Part print with two shaded views. Sizes in mm from the minimum x, y, z corner. A direction names the side the tool comes from. Coordinates: 2 decimals unless noted, no trailing zeros. Write each loop counter-clockwise with the first axis right and the second up, starting at its lowest first coordinate (ties: lowest second). Pieces come first, ordered by that corner, then holes.
Q1. Which spindle directions (+Z, -Z, +X, -X, +Y, -Y) get a long thin tool onto all of the face, cutting with end or side? Do the marked faces 1, 2 and 3. Say none if no direction does.
Q2. Band-saw the part on B-B, the plane y = 17. Write the cut outline in (x, z).
Q3. Drill centre lines: probe 1 along X at (y, z) = (20, 9.25); probe 2 along Z at (x, y) = (22, 26); probe 3 along Z at (x, y) = (30, 13). Where is each one in solid material? Low to high.
Q4. Band-saw the part on A-A, the plane z = 13.5. Write the cut outline in (x, y).
Q5. Pin check, flat tips, straight feed: P1, Ø3, axis at x = 18.5, z = 9, coming from the -Y side; P2, Ø6, axis at y = 24, z = 5.5, coming from the -X side; P3, Ø1.8, axis at y = 16.5, z = 12, coming from the +X side. Stop position of each tip, or through.
Q6. Band-saw the part on C-C, the plane z = 4.5. Write the cut outline in (x, y).
Q7. Band-saw the part on D-D, the plane z = 7.25. Write the cut outline in (x, y).
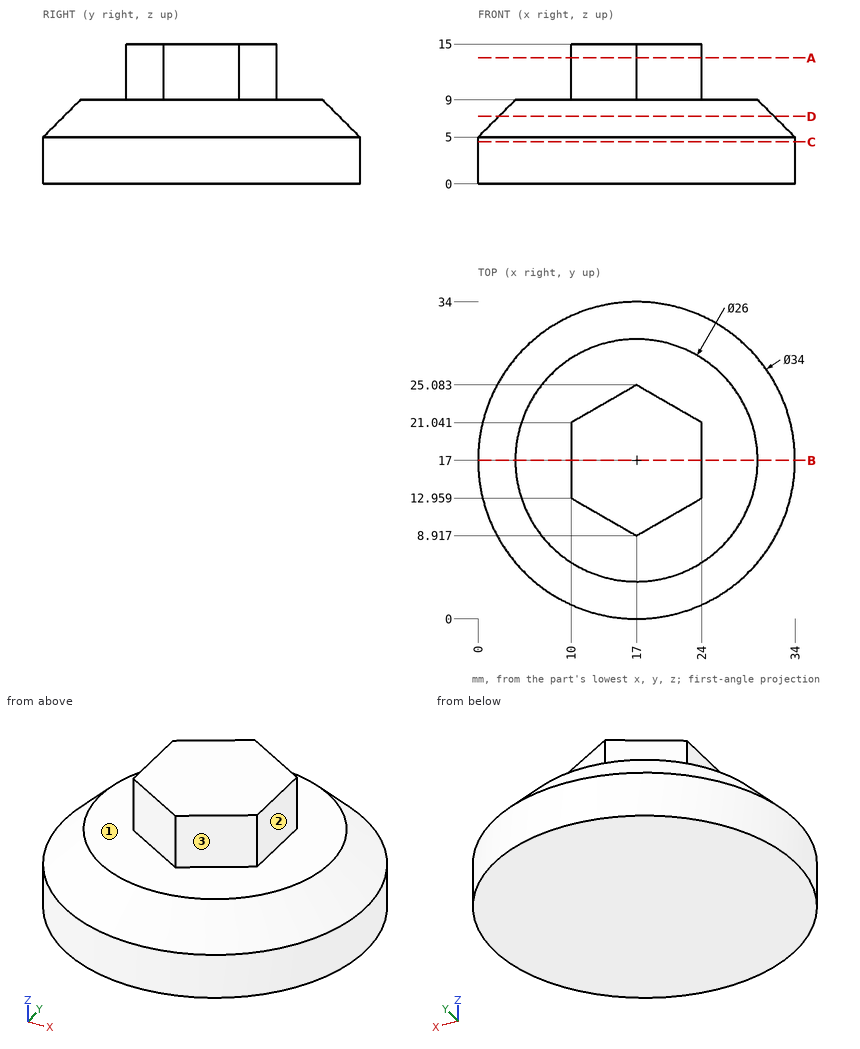
Answer sheet:
1. face 1: +Z
1. face 2: +Z, +X, +Y, -Y
1. face 3: +Z, +X, -Y
2. outline: (0, 0) - (34, 0) - (34, 5) - (30, 9) - (24, 9) - (24, 15) - (10, 15) - (10, 9) - (4, 9) - (0, 5) - close
3. probe 1: x = 10 to 24
3. probe 2: z = 0 to 9
3. probe 3: z = 0 to 8.4
4. outline: (10, 12.96) - (17, 8.92) - (24, 12.96) - (24, 21.04) - (17, 25.08) - (10, 21.04) - close
5. P1: stops at y = 2.57
5. P2: stops at x = 0.49
5. P3: stops at x = 24
6. outline: circle Ø34 at (17, 17)
7. outline: circle Ø29.5 at (17, 17)
